Part print with two shaded views. Sizes in mm from the minimum x, y, z corner. A direction names the side the tool comes from. Coordinates: 2 decimals unless noted, no trailing zeros. Write each loop counter-clockwise with the first axis right and the second up, starting at its lowest first coordinate (ties: lowest second). Pieces come first, ordered by that corner, then holes. Notation, with made-up numbers: (-32.75, 57.5) - (4.25, 57.5) arc R20 ccw to (4.25, 65.5) - close; hole circle Ø1 at (-7.75, -22). An arc over 180 degrees is marked (long way). Answer in a Markdown table with one row per item. Add a question column.
Q1. Band-saw the part on A-A (y = 9). List the corners of the cut face in (x, z), and give its area (3 significant figures).
Q2. 3-axis set-ups, long thin cutter, end or side, ignore diameter. For the marked faces 3 and 4: which of +Z, -Z, +X, -X, +Y, -Y reach the whole face in a straight line?
Q3. Two-plate mould, pull along Y, no slides. Class the marked faces 1 and 2: +Y half, -Y half, draft (parallel to the pull), parting line (faces both ways), or undercut.
Q4. Band-saw the part on C-C (z = 13). List the corners of the cut face in (x, y).
Q5. Drill centre lines: line 1 along X through (y, z) = (9, 2.75); line 2 along Y through (x, z) = (9, 10.75). Where is each one in solid material? Low to high. Write a range as from..to.
Q6. Pin check, flat tips, straight feed: pin 1 (8 mm diameter, centred on y = 4.5, z = 15.5, fed in from -X); pin 2 (2 mm diameter, centred on x = 14.5, z = 22, fed in from +Y); pin 3 (8 mm diameter, centred on x = 9, y = 9, fed in from +Z); pin 4 (6 mm diameter, centred on y = 4.5, z = 22, fed in from +X). Stop position of each tip, or through.
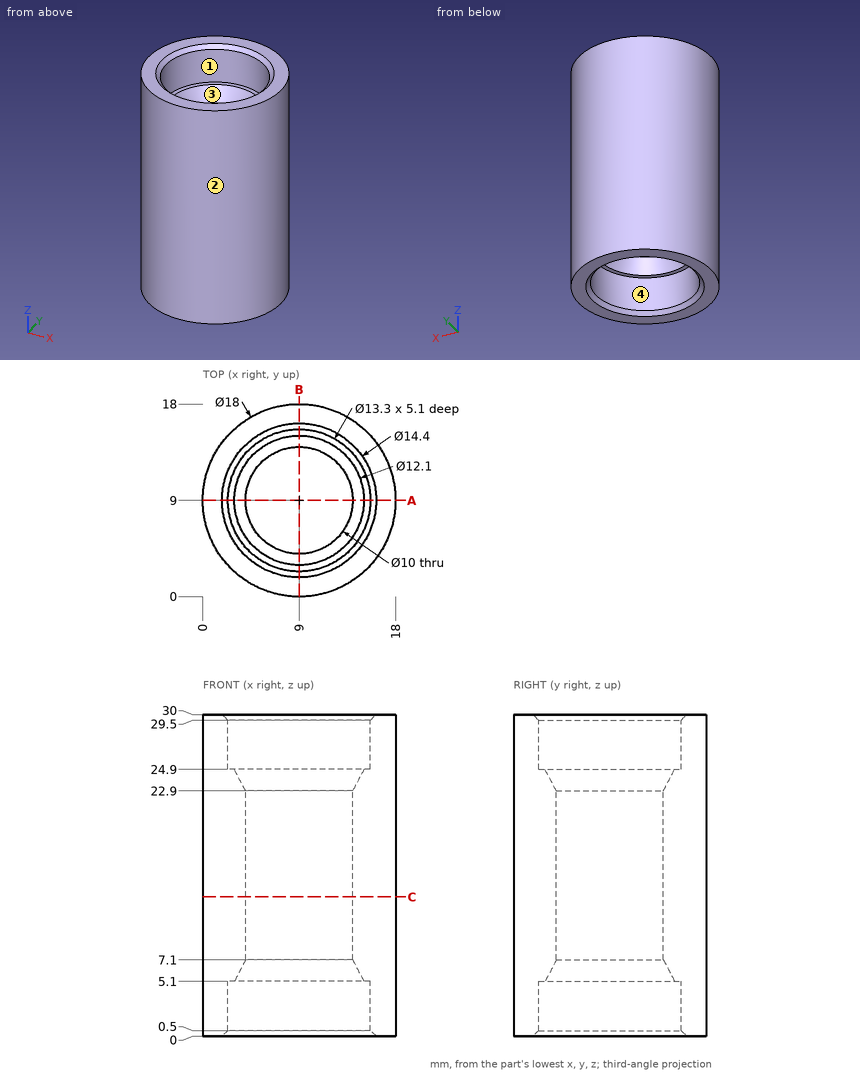
Checked values:
| question | item | result |
|---|---|---|
| 1 | outline | (0, 0) - (1.8, 0) - (2.35, 0.5) - (2.35, 5.1) - (2.95, 5.1) - (4, 7.1) - (4, 22.9) - (2.95, 24.9) - (2.35, 24.9) - (2.35, 29.5) - (1.8, 30) - (0, 30) - close; (14, 7.1) - (15.05, 5.1) - (15.65, 5.1) - (15.65, 0.5) - (16.2, 0) - (18, 0) - (18, 30) - (16.2, 30) - (15.65, 29.5) - (15.65, 24.9) - (15.05, 24.9) - (14, 22.9) - close |
| 1 | area | 202 mm² |
| 2 | face 3 | +Z |
| 2 | face 4 | -Z |
| 3 | face 1 | undercut |
| 3 | face 2 | parting line |
| 4 | outline | circle Ø18 at (9, 9); hole circle Ø10 at (9, 9) |
| 5 | line 1 | x = 0..2.35, 15.65..18 |
| 5 | line 2 | y = 0..4, 14..18 |
| 6 | pin 1 | stops at x = 0.01 |
| 6 | pin 2 | stops at y = 16.79 |
| 6 | pin 3 | passes through |
| 6 | pin 4 | stops at x = 17.87 |
